Can you work these out from the model? Positions are in its coordinate system, mm. A direction names the side the tool comes from. Give positions to 0.01 mm unless a question says otherwise; leave off trailing zeros. Loops run counter-clockwise (first coordinate to the right, second up) from the corner with the lowest first, then second, coordinate; pieces in that order, holes last.
from build123d import *

# Parameters (mm, degrees)
F9_D      = 6.35
F12_R     = 3.175
F13_DEPTH = 25.4


with BuildPart() as f1:
    # F0 (on Front) → F1 (revolve)
    with BuildSketch(Plane.XZ):
        with BuildLine():
            ThreePointArc((0, 127), (89.802561, 89.802561), (127, 0))
            Line((127, 0), (127, -6.35))
            Line((127, -6.35), (133.35, -6.35))
            Line((133.35, -6.35), (133.35, 0))
            Line((133.35, 0), (171.45, 0))
            Line((171.45, 0), (171.45, 6.35))
            Line((171.45, 6.35), (133.198724, 6.35))
            ThreePointArc((133.198724, 6.35), (92.020242, 96.511644), (0, 133.35))
            Line((0, 133.35), (0, 127))
        make_face()
    revolve(axis=Axis((0, 0, 13.31393), (0, 0, 1)))

    # F4 (on Front) → F5 (revolve, cut)
    with BuildSketch(Plane.XZ):
        with BuildLine():
            ThreePointArc((89.802561, 89.802561), (94.185721, 85.19419), (98.332676, 80.372164))
            Line((98.332676, 80.372164), (100.775306, 82.814794))
            Line((100.775306, 82.814794), (103.02037, 80.56973))
            Line((103.02037, 80.56973), (110.363235, 87.912594))
            Line((110.363235, 87.912594), (94.292689, 94.292689))
            Line((94.292689, 94.292689), (89.802561, 89.802561))
        make_face()
    revolve(axis=Axis((92.047625, 0, 92.047625), (0.707107, 0, 0.707107)), mode=Mode.SUBTRACT)

    # F6 (on Front) → F7 (revolve, cut)
    with BuildSketch(Plane.XZ):
        with BuildLine():
            ThreePointArc((-7.9375, 126.75171), (-3.970691, 126.937912), (0, 127))
            Line((0, 127), (0, 133.35))
            ThreePointArc((0, 133.35), (-3.97051, 133.290876), (-7.9375, 133.113555))
            Line((-7.9375, 133.113555), (-7.9375, 126.75171))
        make_face()
    revolve(axis=Axis((0, 0, 130.175), (0, 0, 1)), mode=Mode.SUBTRACT)

    # F9 (through all)
    with Locations(Plane.XY.offset(6.35)):
        with Locations((0, -152.324362)):
            Hole(F9_D / 2)


with BuildPart() as f11:
    # F10 (on Front) → F11 (revolve)
    with BuildSketch(Plane.XZ):
        with BuildLine():
            Line((-133.35, 0), (-171.45, 0))
            Line((-171.45, 0), (-171.45, -6.35))
            Line((-171.45, -6.35), (-142.875, -6.35))
            ThreePointArc((-142.875, -6.35), (-140.629936, -7.279936), (-139.7, -9.525))
            Line((-139.7, -9.525), (-139.7, -15.055494))
            Line((-139.7, -15.055494), (-135.302346, -15.055494))
            ThreePointArc((-135.302346, -15.055494), (-133.212545, -15.840231), (-132.155779, -17.806529))
            ThreePointArc((-132.155779, -17.806529), (-123.729304, -49.732101), (-107.716849, -78.608542))
            Line((-107.716849, -78.608542), (-48.111879, -160.284902))
            ThreePointArc((-48.111879, -160.284902), (-45.388592, -165.608816), (-44.45, -171.514694))
            Line((-44.45, -171.514694), (-44.45, -183.740515))
            ThreePointArc((-44.45, -183.740515), (-44.793731, -187.343013), (-45.812519, -190.815507))
            Line((-45.812519, -190.815507), (-70.758346, -253.180075))
            Line((-70.758346, -253.180075), (-64.862519, -255.538405))
            Line((-64.862519, -255.538405), (-39.916692, -193.173838))
            ThreePointArc((-39.916692, -193.173838), (-38.558308, -188.543846), (-38.1, -183.740515))
            Line((-38.1, -183.740515), (-38.1, -171.514694))
            ThreePointArc((-38.1, -171.514694), (-39.351456, -163.64019), (-42.982505, -156.541638))
            Line((-42.982505, -156.541638), (-102.587475, -74.865278))
            ThreePointArc((-102.587475, -74.865278), (-119.720338, -42.379719), (-126.841151, -6.35))
            Line((-126.841151, -6.35), (-133.35, -6.35))
            Line((-133.35, -6.35), (-133.35, 0))
        make_face()
    revolve(axis=Axis((0, 0, -52.348059), (0, 0, -1)))

    # F12 (on face) → F13 (cut)
    with BuildSketch(Plane.XY):
        with Locations((0, -152.324362)):
            Circle(F12_R)
        with Locations((76.162181, -131.916767)):
            Circle(F12_R)
        with Locations((131.916767, -76.162181)):
            Circle(F12_R)
        with Locations((152.324362, 0)):
            Circle(F12_R)
        with Locations((131.916767, 76.162181)):
            Circle(F12_R)
        with Locations((76.162181, 131.916767)):
            Circle(F12_R)
        with Locations((0, 152.324362)):
            Circle(F12_R)
        with Locations((-76.162181, 131.916767)):
            Circle(F12_R)
        with Locations((-131.916767, 76.162181)):
            Circle(F12_R)
        with Locations((-152.324362, 0)):
            Circle(F12_R)
        with Locations((-131.916767, -76.162181)):
            Circle(F12_R)
        with Locations((-76.162181, -131.916767)):
            Circle(F12_R)
    extrude(amount=-F13_DEPTH, mode=Mode.SUBTRACT)


solid = f11.part
(1) Which directions (+Z, -Z, +X, -X, +Y, -Y) give clear straight access to the entire face, cutting with the end or side of a thin tool? Please do faces 1 (the cylindrical face through (110.86, -85.01, -12.33)), 2 (the conical face through (40.477, -31.036, -156.319)), 3 (the flat face through (118, -49, -6.35)).
Returned:
face 1: -Z
face 2: none
face 3: +Z
(2) Thinking about a two-plate mould opening in Y: for faces 4 (the cylindrical face through (30.235, -23.183, -177.542)), 5 (the flat face through (88, -101, 0)), 6 (the cylindrical face through (-42.397, 13.352, -177.713)), which applies, pulls with the +Y half, pulls with the -Y half, needs draft (parallel to the pull), parting line crosses it, or undercut?
Returned:
face 4: undercut
face 5: needs draft
face 6: parting line crosses it
(3) Will these pins go through, and if not, where does the flat tip stop? P1, Ø12, axis at x = 75, y = -49, coming from the -Z side; P2, Ø10, axis at x = 152.32, y = 0, coming from the -Z side; P3, Ø5, axis at x = 0, y = 152.32, coming from the +Z side; P4, Ø2, axis at x = -59, y = 103, coming from the -Z side.
Returned:
P1: stops at z = -111.67
P2: stops at z = -6.35
P3: passes through
P4: stops at z = -62.68
(4) Please list where these lines run through material, in increasing order: probe 1 along Y at (x, z) = (0, -2.75); probe 2 along Z at (x, y) = (-118.5, -114.5); probe 3 along X at (y, z) = (-23, -132).
Returned:
probe 1: y = -171.45 to -155.5, -149.15 to -133.35, 133.35 to 149.15, 155.5 to 171.45
probe 2: z = -6.35 to 0
probe 3: x = -64.79 to -56.38, 56.38 to 64.79
(5) Suppose I cut it at A-A on z = -89. List the corners of the cut face in (x, y) for me.
Returned:
outline: circle Ø200.27 at (0, 0); hole circle Ø184.54 at (0, 0)
